Here's how the part is built. I have some questions about the finished solid (model axes, mm). A direction names the side the tool comes from. Give positions to 0.01 mm unless a question says otherwise; leave off trailing zeros. Order: outer loops, then holes, each group sorted by start corner. A loop starts at its lowest first (then second) coordinate and runs counter-clockwise, first axis right, second up. Notation, with made-up numbers: M 41.5,-37 L 55.5,-37 A19 ccw 55.5,-26 Z; hole C 52,-3 d11. An arc over 180 degrees is marked long. One line per item, written item: value. Start each with the question number.
from build123d import *

# Parameters (mm, degrees)
SKETCH_1_R               = 1.5
EXTRUDE_1_DEPTH          = 3
FILLET_5_R               = 4
EXTRUDE_START            = -3
EXTRUDE_2_DEPTH          = 3
FILLET_7_R               = 3
FILLET_8_R               = 10
SKETCH_3_R               = 1.5
CUT_EXTRUDE_1_DEPTH      = 247.206358511
FILLET_9_R               = 3
CUT_EXTRUDE_2_DEPTH      = 9.5
FILLET_10_R              = 3
CUT_EXTRUDE_3_DEPTH      = 9.5
CUT_EXTRUDE_4_DEPTH      = 247.206358511
SKETCH_7_R               = 3.5
SKETCH_7_R_2             = 1.5
CUT_EXTRUDE_5_DEPTH      = 55
SKETCH_8_R               = 6
SKETCH_8_R_2             = 3.5
EXTRUDE_3_DEPTH          = 3
EXTRUDE_5_DEPTH          = 3
CUT_EXTRUDE_6_DEPTH      = 247.206358511
CUT_EXTRUDE_6_DEPTH_BACK = 247.206358511
SKETCH_12_R              = 3.5
FILLET_13_R              = 3
EXTRUDE_6_DEPTH          = 3
FILLET_14_R              = 3
FILLET_15_R              = 15


with BuildPart() as part:
    # 草图1 → 凸台-拉伸1 (new body)
    with BuildSketch(Plane.XY):
        with BuildLine():
            Line((4, -6.5), (4, 17.450012814))
            ThreePointArc((4, 17.450012814), (-70.193717354, 87.672930243), (-44, 186.414284285))
            Line((-44, 186.414284285), (-44, 231.414284285))
            Line((-44, 231.414284285), (-54, 231.414284285))
            Line((-54, 231.414284285), (-54, 190.498344353))
            ThreePointArc((-54, 190.498344353), (-80.042429579, 85.759563462), (-4, 9.169947557))
            Line((-4, 9.169947557), (-4, -6.5))
            ThreePointArc((-4, -6.5), (0, -14.5), (4, -6.5))
        make_face()
        with BuildLine():
            ThreePointArc((-1.5, -9.5), (0, -8), (1.5, -9.5))
            Line((1.5, -9.5), (-1.5, -9.5))
        make_face(mode=Mode.SUBTRACT)
        with Locations((0, 9.5)):
            Circle(SKETCH_1_R, mode=Mode.SUBTRACT)
    extrude(amount=EXTRUDE_1_DEPTH)

    # 圆角5
    fillet_5_edges = [part.edges().sort_by_distance(p)[0] for p in [
        (-54, 190.498344353, 1.5),
        (-54, 231.414284285, 1.5),
        (-44, 186.414284285, 1.5),
    ]]
    fillet(fillet_5_edges, radius=FILLET_5_R)

    # 草图2 → 凸台-拉伸2 (add)
    with BuildSketch(Plane.XY.offset(3).offset(EXTRUDE_START)):
        with BuildLine():
            Line((-45, -14.5), (0, -14.5))
            ThreePointArc((0, -14.5), (-4.472135955, -11.736067977), (-4, -6.5))
            Line((-4, -6.5), (-39, -6.5))
            Line((-39, -6.5), (-55.777803301, 41.431046717))
            ThreePointArc((-55.777803301, 41.431046717), (-66.906324005, 56.106749454), (-75.43024107, 72.433508525))
            Line((-75.43024107, 72.433508525), (-45, -14.5))
        make_face()
    extrude(amount=EXTRUDE_2_DEPTH)

    # 圆角7
    fillet_7_edges = [part.edges().sort_by_distance(p)[0] for p in [
        (-55.777803301, 41.431046717, 1.5),
    ]]
    fillet(fillet_7_edges, radius=FILLET_7_R)

    # 圆角8
    fillet_8_edges = [part.edges().sort_by_distance(p)[0] for p in [
        (-39, -6.5, 1.5),
        (-45, -14.5, 1.5),
    ]]
    fillet(fillet_8_edges, radius=FILLET_8_R)

    # 草图3 → 切除-拉伸1 (cut, through all)
    with BuildSketch(Plane.XY.offset(3)):
        with Locations((0, -9.5)):
            Circle(SKETCH_3_R)
    extrude(amount=-CUT_EXTRUDE_1_DEPTH, mode=Mode.SUBTRACT)

    # 圆角9
    fillet_9_edges = [part.edges().sort_by_distance(p)[0] for p in [
        (4, -6.5, 1.5),
        (-4, -6.5, 1.5),
    ]]
    fillet(fillet_9_edges, radius=FILLET_9_R)

    # 草图4 → 切除-拉伸2 (cut)
    with BuildSketch(Plane.XY.offset(3)):
        with BuildLine():
            Line((-34, -8.5), (-39.133974596, -8.5))
            Line((-39.133974596, -8.5), (-41.700961894, -4.053847577))
            ThreePointArc((-41.700961894, -4.053847577), (-43.75, -3.504809472), (-44.299038106, -5.553847577))
            Line((-44.299038106, -5.553847577), (-40.866025404, -11.5))
            Line((-40.866025404, -11.5), (-34, -11.5))
            ThreePointArc((-34, -11.5), (-32.5, -10), (-34, -8.5))
        make_face()
    extrude(amount=-CUT_EXTRUDE_2_DEPTH, mode=Mode.SUBTRACT)

    # 圆角10
    fillet_10_edges = [part.edges().sort_by_distance(p)[0] for p in [
        (-40.866025404, -11.5, 1.5),
        (-39.133974596, -8.5, 1.5),
    ]]
    fillet(fillet_10_edges, radius=FILLET_10_R)

    # 草图5 → 切除-拉伸3 (cut)
    with BuildSketch(Plane.XY.offset(3)):
        with BuildLine():
            Line((-58.126234927, 178.788922212), (-62.714846418, 172.235705858))
            ThreePointArc((-62.714846418, 172.235705858), (-62.346483006, 170.146613137), (-60.257390285, 170.514976549))
            Line((-60.257390285, 170.514976549), (-55.668778794, 177.068192903))
            ThreePointArc((-55.668778794, 177.068192903), (-56.037142206, 179.157285624), (-58.126234927, 178.788922212))
        make_face()
        with BuildLine():
            Line((-79.5, 119), (-79.5, 111))
            ThreePointArc((-79.5, 111), (-78, 109.5), (-76.5, 111))
            Line((-76.5, 111), (-76.5, 119))
            ThreePointArc((-76.5, 119), (-78, 120.5), (-79.5, 119))
        make_face()
        with BuildLine():
            Line((-62.714846418, 57.764294142), (-58.126234927, 51.211077788))
            ThreePointArc((-58.126234927, 51.211077788), (-56.037142206, 50.842714376), (-55.668778794, 52.931807097))
            Line((-55.668778794, 52.931807097), (-60.257390285, 59.485023451))
            ThreePointArc((-60.257390285, 59.485023451), (-62.346483006, 59.853386863), (-62.714846418, 57.764294142))
        make_face()
    extrude(amount=-CUT_EXTRUDE_3_DEPTH, mode=Mode.SUBTRACT)

    # 草图6 → 切除-拉伸4 (cut, through all)
    with BuildSketch(Plane.XY.offset(3)):
        with BuildLine():
            Line((-49, 219.414284285), (-49, 227.414284285))
            ThreePointArc((-49, 227.414284285), (-47.5, 228.914284285), (-46, 227.414284285))
            Line((-46, 227.414284285), (-46, 219.414284285))
            ThreePointArc((-46, 219.414284285), (-47.5, 217.914284285), (-49, 219.414284285))
        make_face()
    extrude(amount=-CUT_EXTRUDE_4_DEPTH, mode=Mode.SUBTRACT)

    # 草图7 → 切除-拉伸5 (cut)
    with BuildSketch(Plane(origin=(0, 0, 0), x_dir=(-1, 0, 0), z_dir=(0, 0, -1))):
        with Locations((0, -9.5)):
            Circle(SKETCH_7_R)
        with Locations((0, -9.5)):
            Circle(SKETCH_7_R_2, mode=Mode.SUBTRACT)
    extrude(amount=-CUT_EXTRUDE_5_DEPTH, mode=Mode.SUBTRACT)

    # 草图8 → 凸台-拉伸3 (add)
    with BuildSketch(Plane(origin=(0, 0, 0), x_dir=(-1, 0, 0), z_dir=(0, 0, -1))):
        with Locations((0, -9.5)):
            Circle(SKETCH_8_R)
        with Locations((0, -9.5)):
            Circle(SKETCH_8_R_2, mode=Mode.SUBTRACT)
    extrude(amount=-EXTRUDE_3_DEPTH)

    # 草图11 → 凸台-拉伸5 (add)
    with BuildSketch(Plane(origin=(0, 0, 0), x_dir=(-1, 0, 0), z_dir=(0, 0, -1))):
        Polygon((-4, 17.450012814), (-4, -5.027864045), (-6, -9.5), align=None)
        Polygon((4, -3.5), (4, 9.169947557), (7.464101615, 11.169947557), align=None)
    extrude(amount=-EXTRUDE_5_DEPTH)

    # 草图12 → 切除-拉伸6 (cut, two sides: drawn at the far end of the back side and taken through both)
    with BuildSketch(Plane(origin=(0, 0, 0), x_dir=(-1, 0, 0), z_dir=(0, 0, -1)).offset(-CUT_EXTRUDE_6_DEPTH_BACK)):
        with Locations((0, 9.5)):
            Circle(SKETCH_12_R)
    extrude(amount=CUT_EXTRUDE_6_DEPTH + CUT_EXTRUDE_6_DEPTH_BACK, mode=Mode.SUBTRACT)

    # 圆角13
    fillet_13_edges = [part.edges().sort_by_distance(p)[0] for p in [
        (-3.31662479, -14.5, 1.5),
    ]]
    fillet(fillet_13_edges, radius=FILLET_13_R)

    # 草图13 → 凸台-拉伸6 (add)
    with BuildSketch(Plane.XY.offset(3)):
        with BuildLine():
            ThreePointArc((8.899590088, 9.5), (7.576313883, 14.169279569), (4, 17.450012814))
            Line((4, 17.450012814), (5.129683944, 2.227514429))
            ThreePointArc((5.129683944, 2.227514429), (7.901100813, 5.404232712), (8.899590088, 9.5))
        make_face()
    extrude(amount=-EXTRUDE_6_DEPTH)

    # 圆角14
    fillet_14_edges = [part.edges().sort_by_distance(p)[0] for p in [
        (4, 17.450012814, 1.5),
        (5.129683944, 2.227514429, 1.5),
    ]]
    fillet(fillet_14_edges, radius=FILLET_14_R)

    # 圆角15
    fillet_15_edges = [part.edges().sort_by_distance(p)[0] for p in [
        (-7.219978098, 10.136121304, 1.5),
    ]]
    fillet(fillet_15_edges, radius=FILLET_15_R)


solid = part.part
Item 1: We'd pull the mould along Y, two halves only. Please class faces 1 (the face through (-37.762, -4.606, 1.521)), 2 (the face through (-62, 63, 0)), 3 (the face through (-82.213, 134.749, 1.479)): +Y half, -Y half, draft (parallel to the pull), parting line (faces both ways), or undercut.
Item 2: Will these pins go through, and if not, where does the flat tip stop? P1, Ø1.5, axis at x = -36.5, z = 2, coming from the -Y side; P2, Ø1, axis at y = 31, z = 2, coming from the -X side; P3, Ø0.9, axis at y = 223.5, z = 1, coming from the -X side; P4, Ø6.5, axis at x = 0, y = -9.5, coming from the +Z side.
Item 3: I want a section at C-C on y = 159.5. Write out the boundary of the cut face in (x, z), plus the area to 3 significant figures.
Item 4: I want a section at A-A on x = -28.5. Write out the boundary of the cut face in (y, z), plus the area to 3 significant figures.
Item 5: I want a section at D-D on y = 215. Write out the boundary of the cut face in (x, z).
Item 6: Please list where these lines run through material, in increasing order: probe 1 along Y at (x, z) = (0, 2.05); probe 2 along Y at (x, z) = (-37.5, 0.3); probe 3 along X at (y, z) = (-3.5, 2.5). Write a range as [from, to].
Item 7: I want a section at B-B on z = 0.55. Count the separate pieces of the cut face and the enclosed holes in it, plus the area to 3 significant figures.
Item 8: For faces 4 (the face through (-46.347, 14.488, 1.479)), 5 (the face through (-61.584, 32.876, 1.479)), which set-ups out of +Z, -Z, +X, -X, +Y, -Y let a thin tool reach every point of the face, with its end or its side?
Answer below:
1. face 1: undercut
1. face 2: draft
1. face 3: parting line
2. P1: stops at y = -14.5
2. P2: stops at x = -61.1
2. P3: stops at x = -54
2. P4: passes through
3. outline: M -74.6,0 L -63.55,0 L -63.55,3 L -74.6,3 Z
3. area: 33.1 mm²
4. outline: M -14.5,0 L -6.5,0 L -6.5,3 L -14.5,3 Z; M 19.45,0 L 31.16,0 L 31.16,3 L 19.45,3 Z
4. area: 59.1 mm²
5. outline: M -54,0 L -44,0 L -44,3 L -54,3 Z
6. probe 1: y = [-15.5, -13], [-6, 6], [13, 18.44]
6. probe 2: y = [-14.5, -11.5], [-8.5, -4.79], [25.18, 37.75]
6. probe 3: x = [-48.85, -43.74], [-42.26, -39.05], [-4, 5.55]
7. separate pieces: 1
7. enclosed holes: 8
7. area: 3,610 mm²
8. face 4: +Z, -Z
8. face 5: +Z, -Z, -X, -Y
